For this review, take the finished solid that the model builds, in its own axes (mm). A direction names the side the tool comes from. Coordinates: 2 decimals unless noted, no trailing zeros. Write each loop counter-clockwise with the first axis right and the second up, starting at its lowest first coordinate (ties: lowest second). Pieces come first, ordered by that corner, then holes. Notation, with made-up numbers: (5.25, 36.5) - (42.25, 36.5) arc R22 ccw to (42.25, 51.5) - close; hole circle Ø10 at (26.25, -7). An arc over 180 degrees is marked (long way). Write each question's results on one line, items separated by ' | '.
Autodesk Inventor part; units mm, degrees
ref_plane "YZ Plane" through (0, 0, 0) normal (1, 0, 0) x (0, 1, 0)
ref_plane "XZ Plane" through (0, 0, 0) normal (0, 1, 0) x (-1, 0, 0)
ref_plane "XY Plane" through (0, 0, 0) normal (0, 0, 1) x (1, 0, 0)
sketch "Sketch3" plane through (0, 0, 0) normal (0, 0, 1) x (1, 0, 0)
  line L0 (-16.4175, -19.05) -> (15.5825, -19.05)
  line L1 (18.3411, -15.8973) -> (18.3411, 16.1027)
  line L2 (14.9996, 19.05) -> (-17.0004, 19.05)
  line L3 (-19.7589, 15.8973) -> (-19.7589, -16.1027)
  line L4 (-17.0004, 19.05) -> (-19.7589, 15.8973)
  line L5 (14.9996, 19.05) -> (18.3411, 16.1027)
  line L6 (18.3411, -15.8973) -> (15.5825, -19.05)
  line L7 (-19.7589, -16.1027) -> (-16.4175, -19.05)
  line L8 (-5.7625, -10.525) -> (5.7625, -10.525)
  line L9 (5.7625, -10.525) -> (5.7625, 10.525)
  line L10 (5.7625, 10.525) -> (-5.7625, 10.525)
  line L11 (-5.7625, 10.525) -> (-5.7625, -10.525)
  circle A0 centre (-14.25, 13.21) radius 2.045
  circle A1 centre (14.25, 13.21) radius 2.045
  circle A2 centre (-14.25, -13.21) radius 2.045
  circle A3 centre (14.25, -13.21) radius 2.045
  point P0 (0, 0)
  dimension "d10" = 11.525
  dimension "d11" = 21.05
  dimension "d12" = 4.09
  dimension "d13" = 4.09
  dimension "d17" = 4.09
  dimension "d19" = 28.5
  dimension "d21" = 4.09
  dimension "d38" = 10.525
  dimension "d39" = 5.7625
  dimension "d45" = 38.1
  dimension "d46" = 38.1
  dimension "d47" = 32
  dimension "d48" = 32
  dimension "d49" = 32
  dimension "d50" = 32
  dimension "d63" = 28.5
  dimension "d67" = 19.05
  dimension "d68" = 14.25
  dimension "d69" = 14.25
  dimension "d70" = 26.42
  dimension "d72" = 13.21
  dimension "d73" = 26.42
  dimension "d75" = 13.21
extrude "Extrusion5" add sketch "Sketch3" along normal blind 4
properties part number "WG17FLANGE"
Q1. Take a section at B-B on x = 14.25. State the section outline as (y, z) points (3 decimals), plus the area to 3 significant figures.
Results found:
outline: (-19.05, 0) - (-15.255, 0) - (-15.255, 4) - (-19.05, 4) - close; (-11.165, 0) - (11.165, 0) - (11.165, 4) - (-11.165, 4) - close; (15.255, 0) - (19.05, 0) - (19.05, 4) - (15.255, 4) - close | area: 120 mm2
Q2. For pin 1 (4.5 mm diameter, centred on x = -14.25, y = 13.21, fed in from +Z), flat-tipped, find the tip position at first contact; note if it passes through.
Results found:
pin 1: z = 4
Q3. Mouldability with a two-part tool opening along X and no side actions: class faces 1 (the face through (-19.759, 0, 2)), 2 (the face through (-1, 19.05, 2)), 3 (the face through (5.762, 0, 2)) as pulls with the +X half, pulls with the -X half, needs draft (parallel to the pull), parting line crosses it, or undercut.
Results found:
face 1: pulls with the -X half | face 2: needs draft | face 3: undercut
Q4. Take a section at D-D on x = -1. State the section outline as (y, z) points (3 decimals), plus the area to 3 significant figures.
Results found:
outline: (-19.05, 0) - (-10.525, 0) - (-10.525, 4) - (-19.05, 4) - close; (10.525, 0) - (19.05, 0) - (19.05, 4) - (10.525, 4) - close | area: 68.2 mm2
Q5. For faces 4 (the face through (-5.762, 0, 2)), 5 (the face through (16.98, -17.45, 1.97)), list the 3-axis set-ups (+Z, -Z, +X, -X, +Y, -Y) from which the entire face can be reached by the end or side of a thin tool; tool diameter is ignored.
Results found:
face 4: +Z, -Z | face 5: +Z, -Z, +X, -Y
Q6. Take a section at C-C on z = 1.6. State how many separate pieces and enclosed holes the cut face has, plus the area to 3 significant figures.
Results found:
separate pieces: 1 | enclosed holes: 5 | area: 1,140 mm2
Q7. Take a section at A-A on y = 13.21. State the section outline as (x, z) points (3 decimals).
Results found:
outline: (-19.759, 0) - (-16.295, 0) - (-16.295, 4) - (-19.759, 4) - close; (-12.205, 0) - (12.205, 0) - (12.205, 4) - (-12.205, 4) - close; (16.295, 0) - (18.341, 0) - (18.341, 4) - (16.295, 4) - close
Q8. Wall thickness on line 1 along Y through (x, z) = (14.25, 1.35) (3 decimals); line 2 along Y through (x, z) = (4.5, 0.9) (3 decimals); line 3 along X through (y, z) = (-5, 0.35): over which ranges is each line inside the solid? List them lowest first. Write a range as from..to.
Results found:
line 1: -19.05..-15.255, -11.165..11.165, 15.255..19.05 | line 2: -19.05..-10.525, 10.525..19.05 | line 3: -19.76..-5.76, 5.76..18.34
